Autodesk Inventor part; units mm, degrees
ref_plane "YZ Plane" through (0, 0, 0) normal (1, 0, 0) x (0, 1, 0)
ref_plane "XZ Plane" through (0, 0, 0) normal (0, 1, 0) x (-1, 0, 0)
ref_plane "XY Plane" through (0, 0, 0) normal (0, 0, 1) x (1, 0, 0)
sketch "草圖1" plane through (0, 0, 0) normal (0, 0, 1) x (0, 1, 0)
  line L0 (-110, 48) -> (70, 48)
  line L1 (70, 48) -> (70, -502)
  line L2 (70, -502) -> (-110, -502)
  line L3 (-110, -502) -> (-110, 48)
  line L4 (70, -342) -> (26, -342)
  line L5 (26, -342) -> (26, -422)
  line L6 (26, -422) -> (6, -476.9495)
  line L7 (6, -476.9495) -> (6, -502)
  point P0 (0, 0)
  dimension "d0" = 110
  dimension "d1" = 48
  dimension "d2" = 180
  dimension "d3" = 550
  dimension "d10" = 136
  dimension "d11" = 20
  dimension "d12" = 20
  dimension "d13" = 80
  dimension "d19" = 160
extrude "擠出1" add sketch "草圖1" along normal mid plane 653 contours L0 L1 L4 L5 L6 L7 L2 L3
sketch "草圖2" plane through (0, 0, 0) normal (0, 0, 1) x (0, 1, 0)
  line L0 (70, -90) -> (-110, -90)
  line L1 (-110, 48) -> (70, 48)
  line L2 (70, 48) -> (70, -342)
  line L3 (6, -502) -> (-110, -502)
  line L4 (-110, -502) -> (-110, 48)
  line L5 (70, -103.9214) -> (70, -178.9214)
  line L6 (70, -342) -> (26, -342)
  line L7 (26, -342) -> (26, -422)
  line L8 (26, -422) -> (6, -476.9495)
  line L9 (6, -476.9495) -> (6, -502)
  point P0 (0, 0)
  dimension "d6" = 90
extrude "擠出2" cut sketch "草圖2" along normal mid plane 550 contours L0 L4 L1 L2
sketch "草圖3" plane through (0, 0, 0) normal (0, 0, 1) x (0, 1, 0)
  circle A0 centre (0, 0) radius 13.25
  dimension "d4" = 653
  dimension "d14" = 26.5
extrude "擠出3" cut sketch "草圖3" along normal through all both and the other way through all
equation "\"d7\" = Width"
equation "\"th6\" = T1A_th6"
equation "\"Width\" = T1A_R6_Width"
equation "\"T1A_th6\" = 45deg"
equation "\"T1A_R1\" = 585.5331"
equation "\"T1A_R3\" = 252.3048"
equation "\"T1A_R4\" = 320.6953"
equation "\"T1A_R5\" = 419.3047"
equation "\"T1A_R7\" = -221.7475"
equation "\"T1A_R8\" = 369.2781"
equation "\"T1A_R1_Width\" = 756"
equation "\"T1A_R2_Width\" = 756"
equation "\"T1A_R3_Width\" = 344"
equation "\"T1A_R4_Width\" = 756"
equation "\"T1A_Joint_Width\" = 756"
properties part number "Type 1A R6主滑台:1" material "密度7850的鋼"
Here's how the part is built. I have some questions about the finished solid (model axes, mm). A direction names the side the tool comes from. Coordinates: 2 decimals unless noted, no trailing zeros. Order: outer loops, then holes, each group sorted by start corner. A loop starts at its lowest first (then second) coordinate and runs counter-clockwise, first axis right, second up. Notation, with made-up numbers: (57.25, 17.25) -> (73.25, 17.25) arc R29 cw to (73.25, 39.25) -> close; hole circle Ø7 at (19, -18.5). An arc over 180 degrees is marked (long way). Return JSON: item names as keys, results as strings.
1) I'm going to push flat-ended pins straight in: P1, Ø20, axis at x = 485, z = 16.5, coming from the +Y side; P2, Ø12, axis at y = 35, z = -31, coming from the -X side; P3, Ø24, axis at x = 0, y = 0, coming from the +Z side (1 decimal). Where does each tip first touch, or does it pass through?
Conclusion:
{"P1": "stops at y = 6.71", "P2": "stops at x = 90", "P3": "passes through"}
2) If we section it at D-D on y = -6: List the corners of the cut face in (x, z) for me, plus the area to 3 significant figures.
Conclusion:
{"outline": "(-48, -326.5) -> (-11.81, -326.5) -> (-11.81, -275) -> (-48, -275) -> close; (-48, 275) -> (-11.81, 275) -> (-11.81, 326.5) -> (-48, 326.5) -> close; (11.81, -326.5) -> (502, -326.5) -> (502, 326.5) -> (11.81, 326.5) -> (11.81, 275) -> (90, 275) -> (90, -275) -> (11.81, -275) -> close", "area": "281,000 mm²"}
3) If we section it at C-C on y = -96.5: List the corners of the cut face in (x, z) for me, plus the area to 3 significant figures.
Conclusion:
{"outline": "(-48, -326.5) -> (502, -326.5) -> (502, 326.5) -> (-48, 326.5) -> (-48, 275) -> (90, 275) -> (90, -275) -> (-48, -275) -> close", "area": "283,000 mm²"}
4) If I drill on probe 1 along Y at (x, z) = (0, -294); probe 2 along X at (y, z) = (0, 294); probe 3 along Z at (x, y) = (15.5, -73), over which ranges is the centre line in solid material (lowest first)?
Conclusion:
{"probe 1": "y = -110 to -13.25, 13.25 to 70", "probe 2": "x = -48 to -13.25, 13.25 to 502", "probe 3": "z = -326.5 to -275, 275 to 326.5"}
5) If we section it at A-A on x = 0: List the corners of the cut face in (y, z) for me, plus the area to 3 significant figures.
Conclusion:
{"outline": "(-110, -326.5) -> (-13.25, -326.5) -> (-13.25, -275) -> (-110, -275) -> close; (-110, 275) -> (-13.25, 275) -> (-13.25, 326.5) -> (-110, 326.5) -> close; (13.25, -326.5) -> (70, -326.5) -> (70, -275) -> (13.25, -275) -> close; (13.25, 275) -> (70, 275) -> (70, 326.5) -> (13.25, 326.5) -> close", "area": "15,800 mm²"}
6) On a 3-axis mill with a long thin cutter (end or side, diameter ignored), from which of +Z, -Z, +X, -X, +Y, -Y can I reach the whole of each face in a straight line? I mean faces 5 (the flat face through (-48, -21, 300)), 6 (the flat face through (20, -21, 275)), 7 (the flat face through (342, 48, -5)). Say none if no direction works.
Conclusion:
{"face 5": "+Z, -Z, -X, +Y, -Y", "face 6": "-X, +Y, -Y", "face 7": "+Z, -Z, +X, +Y"}
7) If we section it at B-B on z = 257: List the corners of the cut face in (x, y) for me.
Conclusion:
{"outline": "(90, -110) -> (502, -110) -> (502, 6) -> (476.95, 6) -> (422, 26) -> (342, 26) -> (342, 70) -> (90, 70) -> close"}
8) Thinking about a two-plate mould opening in Z: for faces 1 (the flat face through (223, -21, -326.5)), 2 (the flat face through (489, 6, -5)), 3 (the flat face through (90, -19, -4)), 4 (the flat face through (20, -21, -275)), which applies, +Z half, -Z half, draft (parallel to the pull), parting line (faces both ways), or undercut?
Conclusion:
{"face 1": "-Z half", "face 2": "draft", "face 3": "undercut", "face 4": "undercut"}
